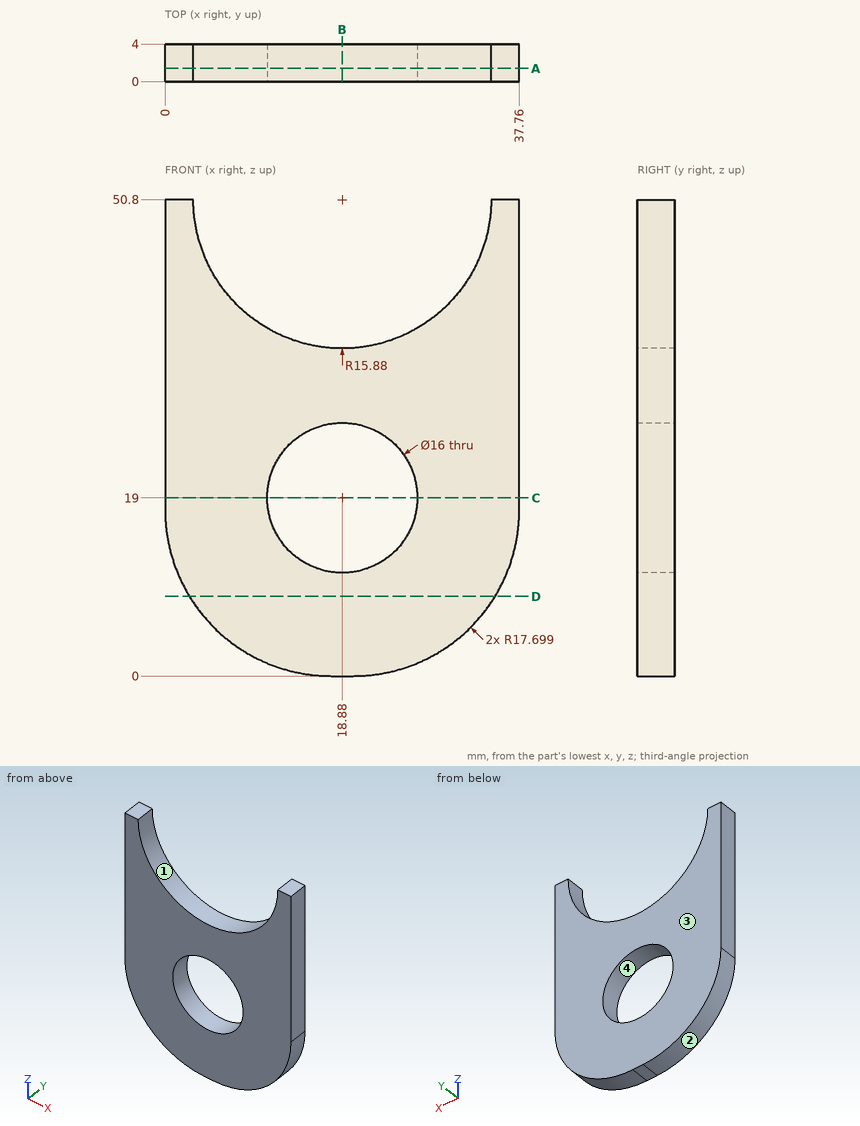
Here's the drawing with two shaded views (mm, measured from the low corner). I have some questions. Round coordinates to 2 decimals unless told otherwise and drop trailing zeros. Order: outer loops, then holes, each group sorted by start corner. A loop starts at its lowest first (then second) coordinate and runs counter-clockwise, first axis right, second up. Notation, with made-up numbers: (75.25, 72) -> (102.25, 72) arc R29 cw to (102.25, 101) -> close; hole circle Ø10 at (63.25, -37.5). An arc over 180 degrees is marked (long way). Use a Markdown table: item, result. Add a question column.
(1) For pin 1 Ø13 at (x, z) = (18.88, 19) entering from -Y; pin 2 Ø1 at (y, z) = (0.5, 33) entering from -X; pin 3 Ø1 at (x, y) = (33, 2.5) entering from +Z; pin 4 Ø1.5 at (x, y) = (13, 1) entering from -Z, each with a flat end and sliding along its axis, tell me the tip position at first contact or that it passes through.
(2) Suppose I cut it at C-C, the plane z = 19. Please give me the cut outline in (x, y), and give its area (3 significant figures).
(3) I need wall thicknesses on line 1 along X through (y, z) = (2.9, 19); line 2 along Z through (x, y) = (19, 3.25); line 3 along X through (y, z) = (2.1, 18). Which ranges of each line are inside material? Lowest first, please.
(4) Suppose I cut it at A-A, the plane y = 1.4. Please give me the cut outline in (x, z), and give its area (3 significant figures).
(5) If we mould it in two halves opening along X, with no side actions, what happens to the marked faces 1, 2, 3 and 4? For each: released by +X, released by -X, zero draft, split by the parting line, or undercut.
(6) Suppose I cut it at D-D, the plane z = 8.5. Please give me the cut outline in (x, y), and give its area (3 significant figures).
(7) Suppose I cut it at B-B, the plane x = 18.88. Please give me the cut outline in (y, z).
Verdict:
| question | item | result |
|---|---|---|
| 1 | pin 1 | through |
| 1 | pin 2 | x = 0 |
| 1 | pin 3 | z = 44.6 |
| 1 | pin 4 | z = 0.45 |
| 2 | outline | (0, 0) -> (10.88, 0) -> (10.88, 4) -> (0, 4) -> close; (26.88, 0) -> (37.76, 0) -> (37.76, 4) -> (26.88, 4) -> close |
| 2 | area | 87.0 mm2 |
| 3 | line 1 | 0 to 10.88, 26.88 to 37.76 |
| 3 | line 2 | 0 to 11, 27 to 34.92 |
| 3 | line 3 | 0 to 10.94, 26.82 to 37.76 |
| 4 | outline | (0, 17.7) arc R17.7 ccw to (17.7, 0) -> (20.06, 0) arc R17.7 ccw to (37.76, 17.7) -> (37.76, 50.8) -> (34.76, 50.8) arc R15.88 cw to (3, 50.8) -> (0, 50.8) -> close; hole circle Ø16 at (18.88, 19) |
| 4 | area | 1,190 mm2 |
| 5 | face 1 | undercut |
| 5 | face 2 | released by -X |
| 5 | face 3 | zero draft |
| 5 | face 4 | undercut |
| 6 | outline | (2.58, 0) -> (35.18, 0) -> (35.18, 4) -> (2.58, 4) -> close |
| 6 | area | 130 mm2 |
| 7 | outline | (0, 0) -> (4, 0) -> (4, 11) -> (0, 11) -> close; (0, 27) -> (4, 27) -> (4, 34.92) -> (0, 34.92) -> close |
